Drawing for the job (mm, zero at the part's lowest x, y, z). A direction names the side the tool comes from. Give positions to 0.01 mm unless a question says otherwise; leave off trailing zeros. Write each loop counter-clockwise with the first axis right and the second up, starting at its lowest first coordinate (ties: lowest second). Pieces come first, ordered by that corner, then holes.
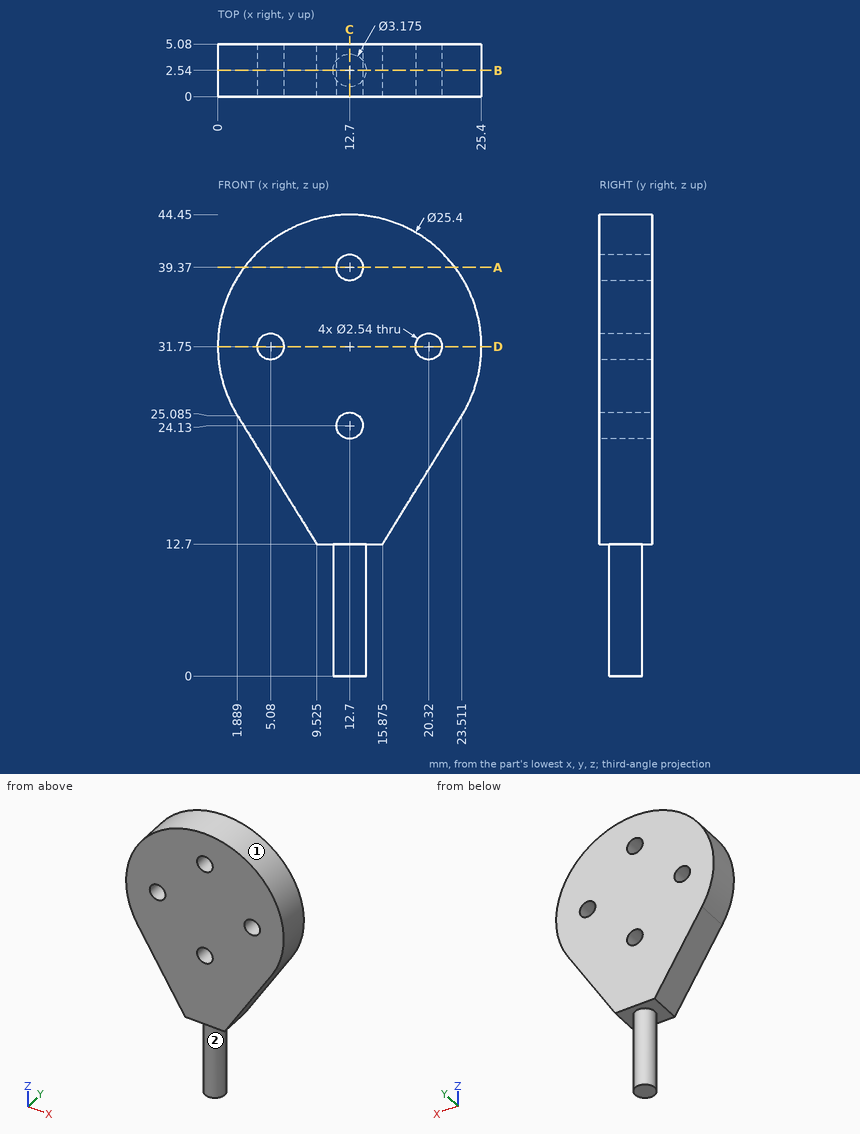
1. Probe probe 1 along X at (y, z) = (2.25, 31.75); probe 2 along X at (y, z) = (2.35, 24.13); probe 3 along X at (y, z) = (1.45, 23) (1 decimal). List the from-to ranges inside material, lowest first.
Calculated:
probe 1: x = 0 to 3.81, 6.35 to 19.05, 21.59 to 25.4
probe 2: x = 2.48 to 11.43, 13.97 to 22.92
probe 3: x = 3.2 to 12.1, 13.3 to 22.2
2. Slice it at C-C, the plane x = 12.7. Write the cut outline in (y, z), and give its area (3 significant figures).
Calculated:
outline: (0, 12.7) - (0.95, 12.7) - (0.95, 0) - (4.13, 0) - (4.13, 12.7) - (5.08, 12.7) - (5.08, 22.86) - (0, 22.86) - close; (0, 25.4) - (5.08, 25.4) - (5.08, 38.1) - (0, 38.1) - close; (0, 40.64) - (5.08, 40.64) - (5.08, 44.45) - (0, 44.45) - close
area: 176 mm2
3. Which spindle directions (+Z, -Z, +X, -X, +Y, -Y) get a long thin tool onto all of the face, cutting with end or side? Do the marked faces 1 and 2. Say none if no direction does.
Calculated:
face 1: +Y, -Y
face 2: -Z
4. Slice it at D-D, the plane z = 31.75. Write the cut outline in (x, y).
Calculated:
outline: (0, 0) - (3.81, 0) - (3.81, 5.08) - (0, 5.08) - close; (6.35, 0) - (19.05, 0) - (19.05, 5.08) - (6.35, 5.08) - close; (21.59, 0) - (25.4, 0) - (25.4, 5.08) - (21.59, 5.08) - close
5. Slice it at B-B, the plane y = 2.54. State how many separate pieces and enclosed holes the cut face has, and give its area (3 significant figures).
Calculated:
separate pieces: 1
enclosed holes: 4
area: 608 mm2
6. Slice it at A-A, the plane z = 39.37. Write the cut outline in (x, y).
Calculated:
outline: (2.54, 0) - (11.43, 0) - (11.43, 5.08) - (2.54, 5.08) - close; (13.97, 0) - (22.86, 0) - (22.86, 5.08) - (13.97, 5.08) - close
7. Pin check, flat tips, straight feed: P1, Ø4, axis at x = 12.7, z = 39.37, coming from the -Y side; P2, Ø3, axis at x = 6.5, y = 3.5, coming from the -Z side (1 decimal); P3, Ø1.5, axis at x = 3, y = 3, coming from the +Z side. Stop position of each tip, or through.
Calculated:
P1: stops at y = 0
P2: stops at z = 15.2
P3: stops at z = 40.76
